Build history of the part. All positions in model axes, mm. Give positions to 0.01 mm unless a question says otherwise; leave off trailing zeros. Loops run counter-clockwise (first coordinate to the right, second up) from the corner with the lowest first, then second, coordinate; pieces in that order, holes last. Notation, with made-up numbers: M 13,-37.5 L 32,-37.5 A22 ccw 32,-13.5 Z; hole C 5.25,58.5 d8. An arc over 180 degrees is marked long. Put each result on its own line as item: value.
```python
from build123d import *

# Parameters (mm, degrees)
SKETCH1_R           = 125.4125
BOSS_EXTRUDE1_DEPTH = 3.175
CUT_EXTRUDE1_DEPTH  = 4.175
CIRPATTERN1_COUNT   = 6
SKETCH3_R           = 15.875
CUT_EXTRUDE2_DEPTH  = 50.8


with BuildPart() as part:
    # Sketch1 → Boss-Extrude1 (new body)
    with BuildSketch(Plane.XY):
        Circle(SKETCH1_R)
    extrude(amount=BOSS_EXTRUDE1_DEPTH)

    # Sketch2 → Cut-Extrude1 (cut, through all)
    with BuildSketch(Plane.XY.offset(3.175)):
        with BuildLine():
            ThreePointArc((93.748147638, 83.304141377), (62.70625, 108.610410952), (25.269428854, 122.840348101))
            add(Edge.make_bspline(
                [(93.748147638, 83.304141377), (15.206576878, 26.338563761), (25.269428854, 122.840348101)],
                knots=[0, 0, 0, 1, 1, 1], degree=2))
        make_face()
    cut_extrude1 = extrude(amount=-CUT_EXTRUDE1_DEPTH, mode=Mode.SUBTRACT)

    # CirPattern1: Cut-Extrude1 ×6 about axis
    cirpattern1_axis = Axis((0, 0, 3.175), (0, 0, -1))
    for i in range(1, CIRPATTERN1_COUNT):
        add(cut_extrude1.rotate(cirpattern1_axis, i * 360 / CIRPATTERN1_COUNT), mode=Mode.SUBTRACT)

    # Sketch3 → Cut-Extrude2 (cut)
    with BuildSketch(Plane(origin=(0, 0, 0), x_dir=(-1, 0, 0), z_dir=(0, 0, -1))):
        Circle(SKETCH3_R)
    extrude(amount=-CUT_EXTRUDE2_DEPTH, mode=Mode.SUBTRACT)


solid = part.part
```
Q1. Mould opens along Y. For faces 1 (the cylindrical face through (108.788, 62.398, 1.565)), 2 (the cylindrical face through (3.441, -15.497, 1.565)), 3 (the cylindrical face through (-108.788, -62.398, 1.565)) say: pulls with the +Y half, pulls with the -Y half, needs draft (parallel to the pull), parting line crosses it, or undercut.
Here are the results:
face 1: pulls with the +Y half
face 2: undercut
face 3: pulls with the -Y half
Q2. Probe line 1 (X direction, y = -69.5, z = 0.8); line 2 (X direction, y = -67.5, z = 0.9); line 3 (Y direction, x = 78, z = 2). List the from-to ranges inside material, lowest first. Write a range as from..to.
Here are the results:
line 1: -104.39..-71.86, -31.92..31.92, 71.86..104.39
line 2: -105.7..-67.77, -33.7..33.7, 67.77..105.7
line 3: -72.9..-10.77, 10.77..72.9
Q3. Slice it at A-A (x = 0). List the corners of the cut face in (y, z) (1 decimal).
Here are the results:
outline: M -125.4,0 L -15.9,0 L -15.9,3.2 L -125.4,3.2 Z; M 15.9,0 L 125.4,0 L 125.4,3.2 L 15.9,3.2 Z
Q4. Slice it at B-B (y = 45). List the corners of the cut face in (x, z) (3 decimals), and give its area (3 significant figures).
Here are the results:
outline: M -117.061,0 L 117.061,0 L 117.061,3.175 L -117.061,3.175 Z
area: 743 mm²
Q5. Drop flat-ended pins along their axis: pin 1 Ø1 at (y, z) = (-50, 0.5) entering from +X; pin 2 Ø1 at (y, z) = (-41.5, 2.5) entering from -X. Give the stop position or say it passes through.
Here are the results:
pin 1: x = 115.23
pin 2: x = -118.52
